Work out the finished part from the listing and answer in its coordinate system (mm). Face numbers are marked on the shaded views. Round coordinates to 2 decimals unless told otherwise and drop trailing zeros. Loops run counter-clockwise (first coordinate to the right, second up) from the corner with the lowest first, then second, coordinate; pieces in that order, holes last.
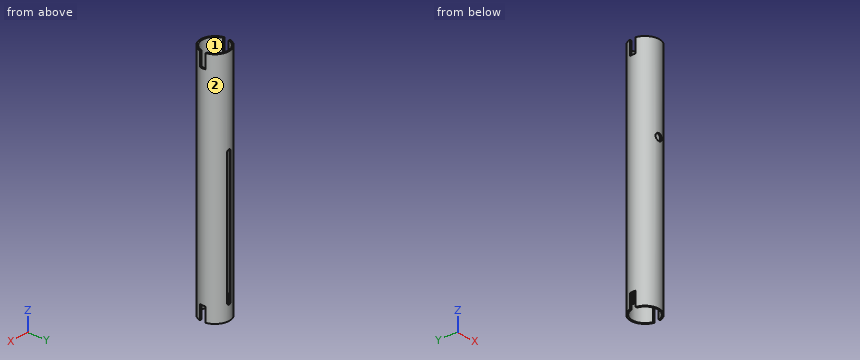
```python
from build123d import *

# Parameters (mm, degrees)
F0_R     = 10
F0_R_2   = 9
F1_DEPTH = 165
F3_DEPTH = 10
F5_DEPTH = 25
F7_DEPTH = 10
F8_R     = 2.5
F9_DEPTH = 25


with BuildPart() as f1:
    # F0 (on Top) → F1 (new body)
    with BuildSketch(Plane.XY):
        Circle(F0_R)
        Circle(F0_R_2, mode=Mode.SUBTRACT)
    extrude(amount=F1_DEPTH)

    # F2 (on Top) → F3 (cut)
    with BuildSketch(Plane.XY):
        with BuildLine():
            ThreePointArc((9.7979589711, -2), (9.9493615301, -1.0050896201), (10, 0))
            ThreePointArc((10, 0), (9.9493615301, 1.0050896201), (9.7979589711, 2))
            Line((9.7979589711, 2), (-9.7979589711, 2))
            ThreePointArc((-9.7979589711, 2), (-10, 0), (-9.7979589711, -2))
            Line((-9.7979589711, -2), (9.7979589711, -2))
        make_face()
    extrude(amount=F3_DEPTH, mode=Mode.SUBTRACT)

    # F4 (on Front) → F5 (cut)
    with BuildSketch(Plane.XZ):
        with BuildLine():
            ThreePointArc((-1.5, 11.5), (0, 10), (1.5, 11.5))
            ThreePointArc((1.5, 11.5), (0, 13), (-1.5, 11.5))
        make_face()
        with BuildLine():
            ThreePointArc((-1.5, 11.5), (0, 13), (1.5, 11.5))
            Line((1.5, 11.5), (1.5, 103.5))
            ThreePointArc((1.5, 103.5), (0, 102), (-1.5, 103.5))
            Line((-1.5, 103.5), (-1.5, 11.5))
        make_face()
        with BuildLine():
            ThreePointArc((-1.5, 103.5), (0, 102), (1.5, 103.5))
            ThreePointArc((1.5, 103.5), (0, 105), (-1.5, 103.5))
        make_face()
    extrude(amount=-F5_DEPTH, mode=Mode.SUBTRACT)

    # F6 (on face) → F7 (cut)
    with BuildSketch(Plane.XY.offset(165)):
        with BuildLine():
            ThreePointArc((10, 0), (9.9493615301, 1.0050896201), (9.7979589711, 2))
            Line((9.7979589711, 2), (8.7749643874, 2))
            ThreePointArc((8.7749643874, 2), (8.9435641521, 1.0063102189), (9, 0))
            ThreePointArc((9, 0), (8.9435641521, -1.0063102189), (8.7749643874, -2))
            Line((8.7749643874, -2), (9.7979589711, -2))
            ThreePointArc((9.7979589711, -2), (9.9493615301, -1.0050896201), (10, 0))
        make_face()
        with BuildLine():
            Line((-8.7749643874, 2), (-9.7979589711, 2))
            ThreePointArc((-9.7979589711, 2), (-10, 0), (-9.7979589711, -2))
            Line((-9.7979589711, -2), (-8.7749643874, -2))
            ThreePointArc((-8.7749643874, -2), (-9, 0), (-8.7749643874, 2))
        make_face()
    extrude(amount=-F7_DEPTH, mode=Mode.SUBTRACT)

    # F8 (on Front) → F9 (cut)
    with BuildSketch(Plane.XZ):
        with Locations((0, 105)):
            Circle(F8_R)
    extrude(amount=F9_DEPTH, mode=Mode.SUBTRACT)


solid = f1.part
```
1. Consider probe 1 along X at (y, z) = (2, 112.5); probe 2 along Z at (x, y) = (0, -9.25). Determine where each line is inside the solid, lowest interval first.
Answer key:
probe 1: x = -9.8 to -8.77, 8.77 to 9.8
probe 2: z = 0 to 102.5, 107.5 to 165
2. Find section B-B (x = 0). Write down the section's boundary in (y, z).
Answer key:
outline: (-10, 0) - (-9, 0) - (-9, 102.5) - (-10, 102.5) - close; (-10, 107.5) - (-9, 107.5) - (-9, 165) - (-10, 165) - close; (9, 0) - (10, 0) - (10, 10) - (9, 10) - close; (9, 105) - (10, 105) - (10, 165) - (9, 165) - close
3. Find section D-D (z = 139.5). Write down the section's boundary in (x, y).
Answer key:
outline: circle Ø20 at (0, 0); hole circle Ø18 at (0, 0)
4. Determine the mould class of the marked faces 1 and 2 for opening direction X: +X half, -X half, draft (parallel to the pull), parting line (faces both ways), or undercut.
Answer key:
face 1: undercut
face 2: parting line
5. Given pin 1 (1.1 mm diameter, centred on x = -9.5, z = 160, fed in from -Y); pin 2 (4 mm diameter, centred on x = -7, z = 102, fed in from +Y); pin 3 (1.1 mm diameter, centred on y = 9.5, z = 66, fed in from +X), each flat-ended and moving along its own axis, determine where each tip first touches the part or whether it passes through.
Answer key:
pin 1: stops at y = -4.46
pin 2: stops at y = 8.66
pin 3: stops at x = 4.46
6. Find section A-A (y = 0). Write down the section's boundary in (x, z), then the cut area to 3 significant figures.
Answer key:
outline: (-10, 10) - (-9, 10) - (-9, 155) - (-10, 155) - close; (9, 10) - (10, 10) - (10, 155) - (9, 155) - close
area: 290 mm2
7. Find section C-C (x = -6.25). Write down the section's boundary in (y, z).
Answer key:
outline: (-7.81, 0) - (-6.48, 0) - (-6.48, 165) - (-7.81, 165) - close; (6.48, 0) - (7.81, 0) - (7.81, 165) - (6.48, 165) - close
